Input: part model. Units: mm. Frame: model coordinates. Face numbers are marked on the shaded views. Coordinates: 2 decimals unless noted, no trailing zeros. Write each loop counter-clockwise with the first axis right and the second up, starting at its lowest first coordinate (ties: lowest second). Pieces come first, ordered by that corner, then holes.
1) Draft query along X for the marked faces 1, 2 and 3. Return one class per face: pulls with the +X half, pulls with the -X half, needs draft (parallel to the pull), parting line crosses it, or undercut.
2) Pin query (flat end, axial travel): pin 1 Ø5 at (x, y) = (-13.86, 8) entering from +Z; pin 2 Ø1.5 at (x, z) = (-10, -12) entering from -Y; pin 3 Ø3.5 at (x, y) = (0, 0) entering from +Z. Return the tip coordinate at first contact, or that it passes through.
3) Line query: L1, parallel to Y at x = -15, z = -12.6; L2, parallel to Y at x = 1, z = -12.1; L3, parallel to Y at x = -0.5, z = -11.3. Output: solid intervals per line, ascending.
4) Section query A-A (y = 0). Output: boundary loops of the cut face in (x, z), then the cut area to 3 significant figures.
5) Section query C-C (z = -10.8). Output: boundary loops of the cut face in (x, y), then the cut area to 3 significant figures.
6) Section query D-D (y = 15). Output: boundary loops of the cut face in (x, z), then the cut area to 3 significant figures.
7) Section query B-B (x = 0). Output: boundary loops of the cut face in (y, z), then the cut area to 3 significant figures.
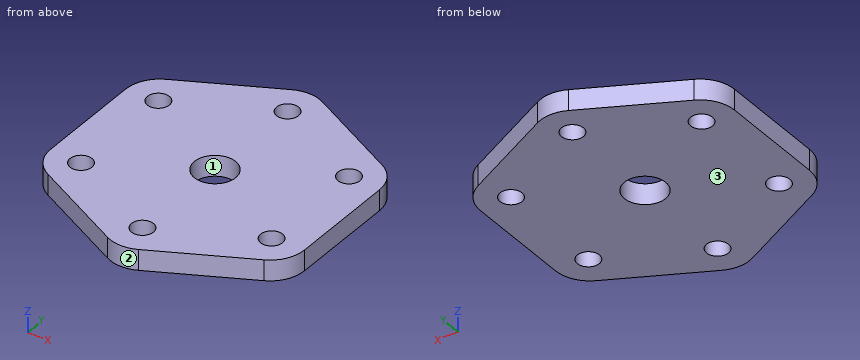
from build123d import *

# Parameters (mm, degrees)
ESBO_O1_R                = 1.6
ESBO_O1_R_2              = 3
RESSALTO_EXTRUS_O1_DEPTH = 3


with BuildPart() as part:
    # Esboço1 → Ressalto-extrusão1 (new body)
    with BuildSketch(Plane(origin=(0, 0, -13), x_dir=(-1, 0, 0), z_dir=(0, 0, -1))):
        with BuildLine():
            Line((-18.456405, 7.753928284), (-18.456405, -7.753928284))
            ThreePointArc((-18.456405, -7.753928284), (-17.715086833, -10.373781151), (-15.710953382, -12.216776208))
            Line((-15.710953382, -12.216776208), (-2.254548382, -19.014703593))
            ThreePointArc((-2.254548382, -19.014703593), (0, -19.551855668), (2.254548382, -19.014703593))
            Line((2.254548382, -19.014703593), (15.710953382, -12.216776208))
            ThreePointArc((15.710953382, -12.216776208), (17.715086833, -10.373781151), (18.456405, -7.753928284))
            Line((18.456405, -7.753928284), (18.456405, 7.753928284))
            ThreePointArc((18.456405, 7.753928284), (17.715086833, 10.373781151), (15.710953382, 12.216776208))
            Line((15.710953382, 12.216776208), (2.254548382, 19.014703593))
            ThreePointArc((2.254548382, 19.014703593), (0, 19.551855668), (-2.254548382, 19.014703593))
            Line((-2.254548382, 19.014703593), (-15.710953382, 12.216776208))
            ThreePointArc((-15.710953382, 12.216776208), (-17.715086833, 10.373781151), (-18.456405, 7.753928284))
        make_face()
        with Locations((13.856405, -8)):
            Circle(ESBO_O1_R, mode=Mode.SUBTRACT)
        with Locations((-13.856405, 8)):
            Circle(ESBO_O1_R, mode=Mode.SUBTRACT)
        with Locations((13.856405, 8)):
            Circle(ESBO_O1_R, mode=Mode.SUBTRACT)
        Circle(ESBO_O1_R_2, mode=Mode.SUBTRACT)
        with Locations((0, 15)):
            Circle(ESBO_O1_R, mode=Mode.SUBTRACT)
        with Locations((-13.856405, -8)):
            Circle(ESBO_O1_R, mode=Mode.SUBTRACT)
        with Locations((0, -15)):
            Circle(ESBO_O1_R, mode=Mode.SUBTRACT)
    extrude(amount=-RESSALTO_EXTRUS_O1_DEPTH)


solid = part.part
Answer:
1. face 1: undercut
1. face 2: parting line crosses it
1. face 3: needs draft
2. pin 1: stops at z = -10
2. pin 2: stops at y = -15.48
2. pin 3: passes through
3. L1: y = -12.58 to -9.12, -6.88 to 6.88, 9.12 to 12.58
3. L2: y = -19.45 to -16.25, -13.75 to -2.83, 2.83 to 13.75, 16.25 to 19.45
3. L3: y = -19.53 to -16.52, -13.48 to -2.96, 2.96 to 13.48, 16.52 to 19.53
4. outline: (-18.46, -13) - (-3, -13) - (-3, -10) - (-18.46, -10) - close; (3, -13) - (18.46, -13) - (18.46, -10) - (3, -10) - close
4. area: 92.7 mm2
5. outline: (-18.46, -7.75) arc R5 ccw to (-15.71, -12.22) - (-2.25, -19.01) arc R5 ccw to (2.25, -19.01) - (15.71, -12.22) arc R5 ccw to (18.46, -7.75) - (18.46, 7.75) arc R5 ccw to (15.71, 12.22) - (2.25, 19.01) arc R5 ccw to (-2.25, 19.01) - (-15.71, 12.22) arc R5 ccw to (-18.46, 7.75) - close; hole circle Ø3.2 at (-13.86, -8); hole circle Ø3.2 at (-13.86, 8); hole circle Ø6 at (0, 0); hole circle Ø3.2 at (0, -15); hole circle Ø3.2 at (0, 15); hole circle Ø3.2 at (13.86, -8); hole circle Ø3.2 at (13.86, 8)
5. area: 1,060 mm2
6. outline: (-10.2, -13) - (-1.6, -13) - (-1.6, -10) - (-10.2, -10) - close; (1.6, -13) - (10.2, -13) - (10.2, -10) - (1.6, -10) - close
6. area: 51.6 mm2
7. outline: (-19.55, -13) - (-16.6, -13) - (-16.6, -10) - (-19.55, -10) - close; (-13.4, -13) - (-3, -13) - (-3, -10) - (-13.4, -10) - close; (3, -13) - (13.4, -13) - (13.4, -10) - (3, -10) - close; (16.6, -13) - (19.55, -13) - (19.55, -10) - (16.6, -10) - close
7. area: 80.1 mm2
